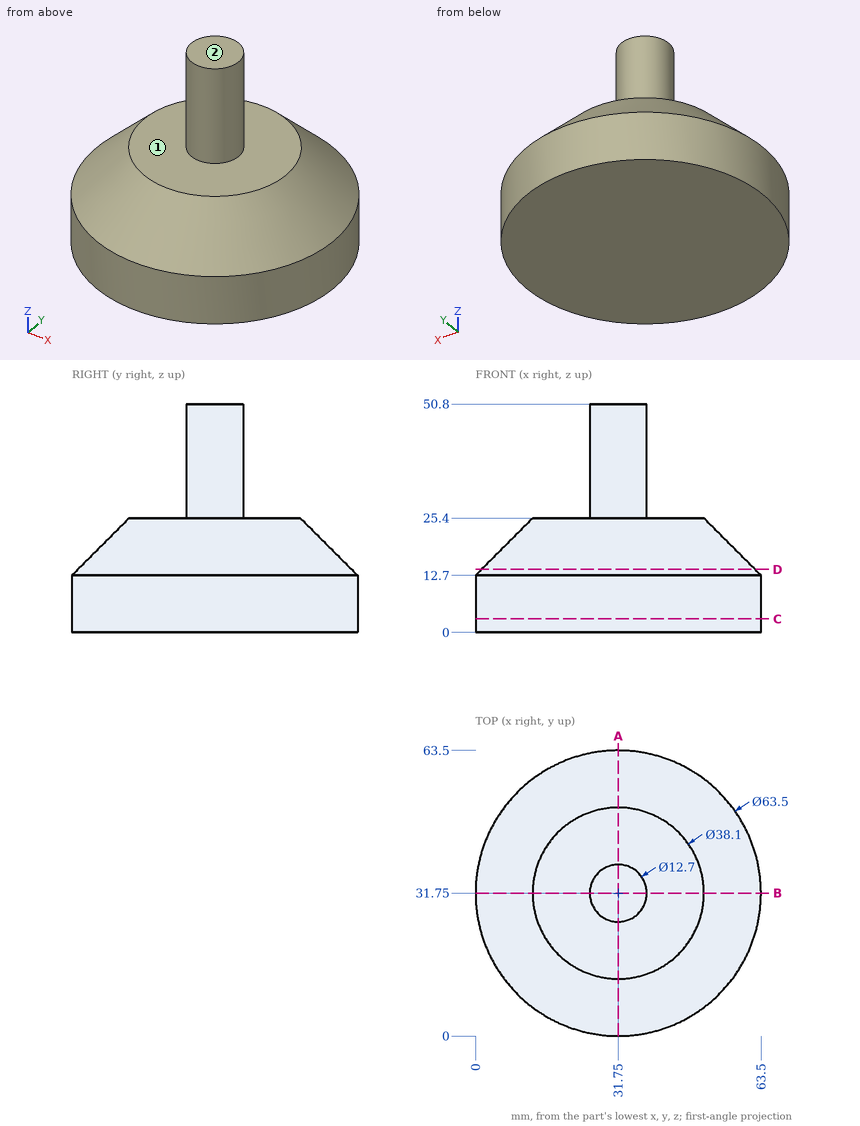
Design review of the part shown in the three views and the two pictorial views. Dimensions are in mm from the part's minimum x, y and z. A direction names the side the tool comes from. Coordinates: 2 decimals unless noted, no trailing zeros. Loops run counter-clockwise (first coordinate to the right, second up) from the corner with the lowest first, then second, coordinate; pieces in that order, holes last. Notation, with made-up numbers: (38, -32) -> (48, -32) arc R33 cw to (48, 1) -> close; hole circle Ø6 at (82, 36.5). An arc over 180 degrees is marked (long way). Answer as CSV lines item,"result".
Item 1: Take a section at D-D, the plane z = 14. State the section outline as (x, y) points, and give its area (3 significant figures).
Results below:
outline,"circle Ø60.9 at (31.75, 31.75)"
area,"2,910 mm2"
Item 2: Take a section at A-A, the plane x = 31.75. State the section outline as (y, z) points.
Results below:
outline,"(0, 0) -> (63.5, 0) -> (63.5, 12.7) -> (50.8, 25.4) -> (38.1, 25.4) -> (38.1, 50.8) -> (25.4, 50.8) -> (25.4, 25.4) -> (12.7, 25.4) -> (0, 12.7) -> close"
Item 3: Take a section at C-C, the plane z = 3. State the section outline as (x, y) points, and give its area (3 significant figures).
Results below:
outline,"circle Ø63.5 at (31.75, 31.75)"
area,"3,170 mm2"
Item 4: Insertion check: pin 1 (5 mm diameter, centred on x = 27, z = 41.5, fed in from +Y); pin 2 (6 mm diameter, centred on x = 38.5, z = 37, fed in from -Y); pin 3 (1.5 mm diameter, centred on y = 36.5, z = 29, fed in from +X). Each pin has a flat end and moves straight along its axis. Give the tip position at first contact, or say it passes through.
Results below:
pin 1,"stops at y = 37.69"
pin 2,"stops at y = 26.63"
pin 3,"stops at x = 36.68"
Item 5: For L1, parallel to X at y = 32.5, z = 7.5; L2, parallel to Z at x = 36.5, y = 27; L3, parallel to X at y = 11, z = 21.5, list the stretches that pass through material, from the lowest coordinate up.
Results below:
L1,"x = 0.01 to 63.49"
L2,"z = 0 to 25.4"
L3,"x = 21.94 to 41.56"
Item 6: Machinability: for the marked faces 1 and 2, which of the approach directions +Z, -Z, +X, -X, +Y, -Y give a long, thin tool a straight path to every point of the face, cutting with its end or side? Answer none if there is none.
Results below:
face 1,"+Z"
face 2,"+Z, +X, -X, +Y, -Y"
